Input: part model. Units: mm. Frame: model coordinates. Coordinates: 2 decimals unless noted, no trailing zeros. Write each loop counter-clockwise with the first axis right and the second up, starting at its lowest first coordinate (ties: lowest second). Pieces come first, ordered by that corner, then holes. Notation, with made-up numbers: (38, 53) -> (61, 53) arc R16 ccw to (61, 62) -> close; hole circle Ø2 at (82, 48.5). An arc over 180 degrees is marked (long way). Use one line per item in the form item = value. Start each with the question number.
(1) Ray query, line 1 along Y through (x, z) = (-66.5, 0); line 2 along X through (y, z) = (-4.5, 2); line 3 along Y through (x, z) = (-72, -1.25). Return the intervals inside material, ascending.
(2) First-contact query: pin 1 (1.5 mm diameter, centred on y = -6.5, z = 0.5, fed in from +X); pin 2 (1.2 mm diameter, centred on x = 117, y = -4.5, fed in from -Z); pin 3 (4.5 mm diameter, centred on x = -115, y = -4.5, fed in from -Z); pin 4 (2 mm diameter, centred on y = -6, z = -2, fed in from +X). Flat tips, straight axial feed; report the tip coordinate or a pass-through.
(3) Cut plane A-A on z = -0.5. Return the cut outline in (x, y).
(4) Cut plane B-B on x = 83.5. Return the cut outline in (y, z).
(5) Pull-direction query (X, two-part tool) for faces 1 (the face through (-2, -2, 0)), 2 (the face through (128, -2, -1)), 3 (the face through (-128, -2, -1)), 4 (the face through (1.79, 2.53, -1.61)); classes: released by +X, released by -X, zero draft, split by the parting line, or undercut.
```python
from build123d import *

# Parameters (mm, degrees)
SKETCH_1_R      = 3
SKETCH_1_R_2    = 2
EXTRUDE_1_DEPTH = 128
EXTRUDE_START   = 10
EXTRUDE_2_DEPTH = 10


with BuildPart() as part:
    # 草圖1 → 填料-伸長1 (new, symmetric)
    with BuildSketch(Plane(origin=(0, 0, 0), x_dir=(0, 0, -1), z_dir=(1, 0, 0))):
        Circle(SKETCH_1_R)
        Circle(SKETCH_1_R_2, mode=Mode.SUBTRACT)
    extrude(amount=EXTRUDE_1_DEPTH, both=True)

    # 草圖2 → 填料-伸長2 (add)
    with BuildSketch(Plane(origin=(110, 0, 0), x_dir=(0, 0, -1), z_dir=(1, 0, 0)).offset(EXTRUDE_START)):
        with BuildLine():
            Line((-3, 0), (-3, -7))
            ThreePointArc((-3, -7), (-1.75, -8.25), (-0.5, -7))
            Line((-0.5, -7), (-0.5, -2.958039892))
            ThreePointArc((-0.5, -2.958039892), (-2.291287847, -1.936491673), (-3, 0))
        make_face()
    extrude_2 = extrude(amount=-EXTRUDE_2_DEPTH)

    # 鏡射1: 填料-伸長2 across plane
    add(extrude_2.mirror(Plane(origin=(0, 0, 0), x_dir=(0, 0, 1), z_dir=(1, 0, 0))))


solid = part.part
```
Values:
q1.line_1 = -3 to -2, 2 to 3
q1.line_2 = -120 to -110, 110 to 120
q1.line_3 = -2.73 to -1.56, 1.56 to 2.73
q2.pin_1 = 120
q2.pin_2 = 0.5
q2.pin_3 = -1.98
q2.pin_4 = through
q3.outline = (-128, -2.96) -> (128, -2.96) -> (128, -1.94) -> (-128, -1.94) -> close; (-128, 1.94) -> (128, 1.94) -> (128, 2.96) -> (-128, 2.96) -> close
q4.outline = circle Ø6 at (0, 0); hole circle Ø4 at (0, 0)
q5.face_1 = zero draft
q5.face_2 = released by +X
q5.face_3 = released by -X
q5.face_4 = undercut
